Build history of the part. All positions in model axes, mm. Face numbers are marked on the shaded views. A direction names the side the tool comes from. Give positions to 0.01 mm unless a question says otherwise; leave off trailing zeros. Order: outer loops, then holes, each group sorted by start corner. A loop starts at its lowest first (then second) coordinate and runs counter-clockwise, first axis right, second up. Notation, with made-up numbers: (55, -18.75) - (88, -18.75) arc R22 cw to (88, -9.75) - close; hole circle Ø9 at (-27, 7.25). An arc over 180 degrees is marked (long way). Use a Markdown table: item, result.
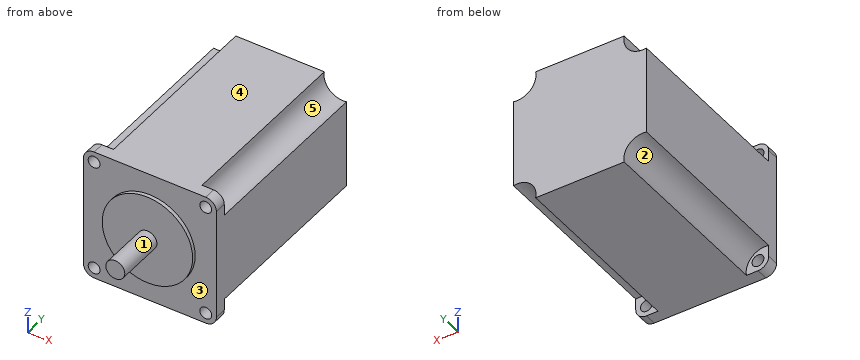
from build123d import *

# Parameters (mm, degrees)
SKETCH_R     = 2.5
PAD_DEPTH    = 5
SKETCH001_R  = 19.05
PAD001_DEPTH = 1.6
SKETCH002_R  = 4
PAD002_DEPTH = 20.5
PAD003_DEPTH = 78


with BuildPart() as part:
    # Sketch → Pad (new body)
    with BuildSketch(Plane.XZ):
        with BuildLine():
            Line((-28, 23.499995), (-28, -23.499995))
            ThreePointArc((-28, -23.499995), (-26.681977, -26.681984), (-23.499985, -28))
            Line((-23.499985, -28), (23.500005, -28))
            ThreePointArc((23.500005, -28), (26.681984, -26.681977), (28, -23.499995))
            Line((28, 23.499995), (28, -23.499995))
            ThreePointArc((28, 23.499995), (26.681981, 26.681981), (23.499995, 28))
            Line((-23.499995, 28), (23.499995, 28))
            ThreePointArc((-23.499995, 28), (-26.681981, 26.681981), (-28, 23.499995))
        make_face()
        with Locations((-23.5, 23.5)):
            Circle(SKETCH_R, mode=Mode.SUBTRACT)
        with Locations((23.5, 23.5)):
            Circle(SKETCH_R, mode=Mode.SUBTRACT)
        with Locations((-23.5, -23.5)):
            Circle(SKETCH_R, mode=Mode.SUBTRACT)
        with Locations((23.5, -23.5)):
            Circle(SKETCH_R, mode=Mode.SUBTRACT)
    extrude(amount=PAD_DEPTH)

    # Sketch001 (on Face14 of Pad) → Pad001 (join)
    with BuildSketch(Plane.XZ.offset(5)):
        Circle(SKETCH001_R)
    extrude(amount=PAD001_DEPTH)

    # Sketch002 (on Face16 of Pad001) → Pad002 (join)
    with BuildSketch(Plane.XZ.offset(6.6)):
        Circle(SKETCH002_R)
    extrude(amount=PAD002_DEPTH)

    # Sketch003 (on Face4 of Pad002) → Pad003 (join)
    with BuildSketch(Plane(origin=(0, 0, 0), x_dir=(1, 0, 0), z_dir=(0, 1, 0))):
        with BuildLine():
            Line((-18.641883, 28), (18.641883, 28))
            ThreePointArc((18.641883, 28), (20.843146, 20.843146), (28, 18.641883))
            Line((28, 18.641883), (28, -18.641883))
            ThreePointArc((28, -18.641883), (20.843146, -20.843146), (18.641883, -28))
            Line((-18.641883, -28), (18.641883, -28))
            ThreePointArc((-18.641883, -28), (-20.843146, -20.843146), (-28, -18.641883))
            Line((-28, -18.641883), (-28, 18.641883))
            ThreePointArc((-28, 18.641883), (-20.843146, 20.843146), (-18.641883, 28))
        make_face()
    extrude(amount=PAD003_DEPTH)


solid = part.part
1) Slice it at B-B (x = 0). Write the cut outline in (y, z), and give its area (3 significant figures).
Computed:
| item | result |
|---|---|
| outline | (-27.1, -4) - (-6.6, -4) - (-6.6, -19.05) - (-5, -19.05) - (-5, -28) - (78, -28) - (78, 28) - (-5, 28) - (-5, 19.05) - (-6.6, 19.05) - (-6.6, 4) - (-27.1, 4) - close |
| area | 4,870 mm² |
2) Slice it at C-C (y = 32). Write the cut outline in (x, z), and give its area (3 significant figures).
Computed:
| item | result |
|---|---|
| outline | (-28, -18.64) arc R8 cw to (-18.64, -28) - (18.64, -28) arc R8 cw to (28, -18.64) - (28, 18.64) arc R8 cw to (18.64, 28) - (-18.64, 28) arc R8 cw to (-28, 18.64) - close |
| area | 2,830 mm² |
3) Tool access for the marked faces 4 and 5: list every direction of +Z, -Z, +X, -X, +Y, -Y with a clear straight run to the whole face (end or side of a thin tool).
Computed:
| item | result |
|---|---|
| face 4 | +Z, +X, -X, +Y, -Y |
| face 5 | +Y |
4) Two-plate mould, pull along X, no slides. Class the marked faces 1, 2 and 3: +X half, -X half, draft (parallel to the pull), parting line (faces both ways), or undercut.
Computed:
| item | result |
|---|---|
| face 1 | parting line |
| face 2 | undercut |
| face 3 | draft |
5) Pin check, flat tips, straight feed: P1, Ø12, axis at x = -1.5, z = -22, coming from the -Y side; P2, Ø6.5, axis at x = -23.5, z = -23.5, coming from the -Y side. Stop position of each tip, or through.
Computed:
| item | result |
|---|---|
| P1 | stops at y = -6.6 |
| P2 | stops at y = -5 |
6) Slice it at A-A (z = 0). Write the cut outline in (x, y).
Computed:
| item | result |
|---|---|
| outline | (-28, -5) - (-19.05, -5) - (-19.05, -6.6) - (-4, -6.6) - (-4, -27.1) - (4, -27.1) - (4, -6.6) - (19.05, -6.6) - (19.05, -5) - (28, -5) - (28, 78) - (-28, 78) - close |
7) Slice it at D-D (z = 16.5). Write the cut outline in (x, y), and give its area (3 significant figures).
Computed:
| item | result |
|---|---|
| outline | (-28, -5) - (-9.52, -5) - (-9.52, -6.6) - (9.52, -6.6) - (9.52, -5) - (28, -5) - (28, 78) - (-28, 78) - close |
| area | 4,680 mm² |
8) Wall check: line 1 (X direction, y = -3, z = -23); line 2 (Y direction, x = 3, z = 13); line 3 (Y direction, x = -20, z = 6). Give the ranges that are in metal, low to high. Write a range as from..to.
Computed:
| item | result |
|---|---|
| line 1 | x = -28..-25.95, -21.05..21.05, 25.95..28 |
| line 2 | y = -6.6..78 |
| line 3 | y = -5..78 |
